from build123d import *

# Parameters (mm, degrees)
SKETCH_1_W          = 28
SKETCH_1_H          = 28
SKETCH_1_W_2        = 13
SKETCH_1_H_2        = 13
EXTRUDE_1_DEPTH     = 5
SKETCH_3_R          = 1.5
CUT_EXTRUDE_1_DEPTH = 40.912404087
SKETCH_6_R          = 1.5
CUT_EXTRUDE_2_DEPTH = 40.912404087


with BuildPart() as part:
    # Эскиз1 → Бобышка-Вытянуть1 (new body)
    with BuildSketch(Plane(origin=(0, 0, 0), x_dir=(1, 0, 0), z_dir=(0, 1, 0))):
        with Locations((14, 14)):
            Rectangle(SKETCH_1_W, SKETCH_1_H)
        with Locations((14, 14)):
            Rectangle(SKETCH_1_W_2, SKETCH_1_H_2, mode=Mode.SUBTRACT)
    extrude(amount=EXTRUDE_1_DEPTH)

    # Эскиз3 → Вырез-Вытянуть1 (cut, through all)
    with BuildSketch(Plane(origin=(0, 5, 0), x_dir=(1, 0, 0), z_dir=(0, 1, 0))):
        with Locations(Location((24, 24, 0), (0, 0, 270))):
            Circle(SKETCH_3_R)
    extrude(amount=-CUT_EXTRUDE_1_DEPTH, mode=Mode.SUBTRACT)

    # Эскиз6 → Вырез-Вытянуть2 (cut, through all)
    with BuildSketch(Plane(origin=(0, 5, 0), x_dir=(1, 0, 0), z_dir=(0, 1, 0))):
        with Locations(Location((4, 24, 0), (0, 0, 270))):
            Circle(SKETCH_6_R)
        with Locations(Location((4, 4, 0), (0, 0, 270))):
            Circle(SKETCH_6_R)
        with Locations(Location((24, 4, 0), (0, 0, 270))):
            Circle(SKETCH_6_R)
        with Locations(Location((24, 14, 0), (0, 0, 270))):
            Circle(SKETCH_6_R)
        with Locations(Location((14, 24, 0), (0, 0, 270))):
            Circle(SKETCH_6_R)
        with Locations(Location((4, 14, 0), (0, 0, 270))):
            Circle(SKETCH_6_R)
        with Locations(Location((14, 4, 0), (0, 0, 270))):
            Circle(SKETCH_6_R)
    extrude(amount=-CUT_EXTRUDE_2_DEPTH, mode=Mode.SUBTRACT)


solid = part.part
Here's how the part is built. I have some questions about the finished solid (model axes, mm). A direction names the side the tool comes from. Give positions to 0.01 mm unless a question says otherwise; leave off trailing zeros. Order: outer loops, then holes, each group sorted by start corner. A loop starts at its lowest first (then second) coordinate and runs counter-clockwise, first axis right, second up. Notation, with made-up numbers: (-13, 85) -> (31, 85) arc R25 cw to (31, 123) -> close; hole circle Ø4 at (31, 74.5). An arc over 180 degrees is marked (long way). One line per item, written item: value. Start each with the question number.
1. Imagine slicing it at A-A, the plane y = 3.1. Count the separate pieces of the cut face and the enclosed holes in it, plus the area to 3 significant figures.
2. For faces 1 (the face through (14, 2, -28)), 2 (the face through (14, 2, -7.5)), which set-ups out of +Z, -Z, +X, -X, +Y, -Y let a thin tool reach every point of the face, with its end or its side?
3. I need wall thicknesses on probe 1 along X at (y, z) = (3.8, -4); probe 2 along X at (y, z) = (0.8, -17.75); probe 3 along Z at (x, y) = (17.25, 1.4). Which ranges of each line are inside material? Lowest first, please. Write a range as from..to.
4. Imagine slicing it at C-C, the plane x = 24. List the corners of the cut face in (y, z) for me, plus the area to 3 significant figures.
5. Imagine slicing it at B-B, the plane z = -16.5. List the corners of the cut face in (x, y) for me, plus the area to 3 significant figures.
6. Imagine slicing it at D-D, the plane z = -4. List the corners of the cut face in (x, y) for me, plus the area to 3 significant figures.
Values follow:
1. separate pieces: 1
1. enclosed holes: 9
1. area: 558 mm2
2. face 1: -Z, +X, -X, +Y, -Y
2. face 2: +Y, -Y
3. probe 1: x = 0..2.5, 5.5..12.5, 15.5..22.5, 25.5..28
3. probe 2: x = 0..7.5, 20.5..28
3. probe 3: z = -28..-20.5, -7.5..0
4. outline: (0, -28) -> (5, -28) -> (5, -25.5) -> (0, -25.5) -> close; (0, -22.5) -> (5, -22.5) -> (5, -15.5) -> (0, -15.5) -> close; (0, -12.5) -> (5, -12.5) -> (5, -5.5) -> (0, -5.5) -> close; (0, -2.5) -> (5, -2.5) -> (5, 0) -> (0, 0) -> close
4. area: 95.0 mm2
5. outline: (0, 0) -> (7.5, 0) -> (7.5, 5) -> (0, 5) -> close; (20.5, 0) -> (28, 0) -> (28, 5) -> (20.5, 5) -> close
5. area: 75.0 mm2
6. outline: (0, 0) -> (2.5, 0) -> (2.5, 5) -> (0, 5) -> close; (5.5, 0) -> (12.5, 0) -> (12.5, 5) -> (5.5, 5) -> close; (15.5, 0) -> (22.5, 0) -> (22.5, 5) -> (15.5, 5) -> close; (25.5, 0) -> (28, 0) -> (28, 5) -> (25.5, 5) -> close
6. area: 95.0 mm2
